The model under review builds one solid part; all positions refer to its coordinate system, in mm. Face numbers are marked on the shaded views. A direction names the side the tool comes from. Give positions to 0.01 mm unless a question says otherwise; leave off trailing zeros. Order: outer loops, then holes, each group sorted by start corner. A loop starts at its lowest first (then second) coordinate and runs counter-clockwise, first axis right, second up. Notation, with made-up numbers: (75, 83.5) - (122, 83.5) arc R12 cw to (122, 99.5) - close; hole circle Ø5 at (32, -23.5). An arc over 180 degrees is marked (long way). Put each result on its own line as item: value.
```python
from build123d import *

# Parameters (mm, degrees)
BOSS_EXTRUDE1_DEPTH = 8
SKETCH4_W           = 60
SKETCH4_H           = 30
BOSS_EXTRUDE2_DEPTH = 3
SKETCH5_R           = 3
CUT_EXTRUDE1_DEPTH  = 68.388900825
CUT_EXTRUDE3_DEPTH  = 61.736204501


# Read off the part's stored shape, not the designer's step: Boss-Extrude1
with BuildPart() as part:
    # Boss-Extrude1 outline → Boss-Extrude1 (new body)
    with BuildSketch(Plane.XY):
        with BuildLine():
            Line((-30, 0), (15, 0))
            add(Edge.make_bspline(
                [(15, 0), (15, -35), (-1.465594932, -45)],
                knots=[0, 0, 0, 1, 1, 1], degree=2))
            Line((-1.465594932, -45), (1.12987064, -49.273588476))
            add(Edge.make_bspline(
                [(20, 0), (20, -0.746108231), (19.988920633, -2.249243802), (19.922237871, -5.16766696), (19.754979798, -8.712103145), (19.418395555, -12.782160754), (18.785639236, -17.973362747), (17.643635897, -24.021456658), (15.683824621, -30.584336804), (13.095918314, -36.449845939), (8.74916419, -43.310162254), (4.437502248, -47.26477457), (1.12987064, -49.273588476)],
                knots=[0, 0, 0, 0, 0.03125, 0.0625, 0.125, 0.1875, 0.25, 0.375, 0.5, 0.625, 0.75, 1, 1, 1, 1], degree=3))
            Line((20, 0), (30, 0))
            Line((30, 0), (30, 5))
            Line((30, 5), (-30, 5))
            Line((-30, 5), (-30, 0))
        make_face()
    extrude(amount=BOSS_EXTRUDE1_DEPTH)

    # Sketch4 → Boss-Extrude2 (add)
    with BuildSketch(Plane(origin=(0, 5, 0), x_dir=(1, 0, 0), z_dir=(0, 1, 0))):
        with Locations((0, -4)):
            Rectangle(SKETCH4_W, SKETCH4_H)
    extrude(amount=BOSS_EXTRUDE2_DEPTH)

    # Sketch5 → Cut-Extrude1 (cut, through all)
    with BuildSketch(Plane(origin=(0, 8, 0), x_dir=(1, 0, 0), z_dir=(0, 1, 0))):
        with Locations(Location((25, -4, 0), (0, 0, 180))):
            Circle(SKETCH5_R)
    extrude(amount=-CUT_EXTRUDE1_DEPTH, mode=Mode.SUBTRACT)

    # Sketch7 → Cut-Extrude3 (cut, through all)
    with BuildSketch(Plane.XY.offset(8)):
        Polygon((-1.465594932, -45), (9.447885747, -41.814579425), (11.582932476, -49.129403534), (0.669451797, -52.314824109), align=None)
    extrude(amount=-CUT_EXTRUDE3_DEPTH, mode=Mode.SUBTRACT)


solid = part.part
```
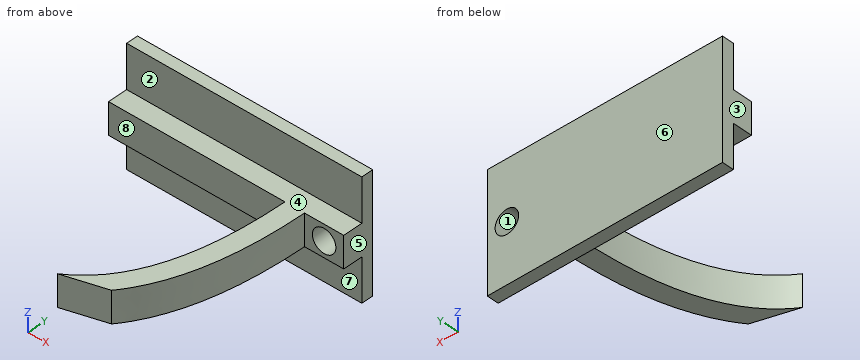
(1) The part is to be moulded in two halves that separate along X. For the marked faces 1, 2 and 3, say which applies: pulls with the +X half, pulls with the -X half, needs draft (parallel to the pull), parting line crosses it, or undercut.
The answers:
face 1: undercut
face 2: needs draft
face 3: pulls with the -X half
(2) Clearance check with flat-ended pins moving along their axes: pin 1 Ø25 at (x, y) = (10, -15.5) entering from +Z; pin 2 Ø3.5 at (x, z) = (2, -7) entering from -Y; pin 3 Ø2.5 at (x, z) = (-16.5, 2.5) entering from -Y. State where each tip first meets the part, or that it passes through.
The answers:
pin 1: z = 8
pin 2: y = 5
pin 3: y = 0
(3) Wall thickness on L1, parallel to Z at x = 25, y = 2.25; L2, parallel to Y at x = -8, z = 16; L3, parallel to X at y = 4, z = 3: over which ranges is each line inside the solid? List them lowest first.
The answers:
L1: 0 to 1, 7 to 8
L2: 5 to 8
L3: -30 to 22.17, 27.83 to 30
(4) For the marked faces 4, 5, 6, 7 and 8, list the 3-axis set-ups (+Z, -Z, +X, -X, +Y, -Y) from which the entire face can be reached by the end or side of a thin tool; tool diameter is ignored.
The answers:
face 4: +Z, +X, -X, -Y
face 5: +Z, -Z, +X, +Y, -Y
face 6: +Z, -Z, +X, -X, +Y
face 7: -Z, +X, -X, -Y
face 8: +Z, -Z, -X
(5) Take a section at C-C, the plane x = -3.5. Write out the cut boundary in (y, z), then the cut area to 3 significant figures.
The answers:
outline: (0, 0) - (5, 0) - (5, -11) - (8, -11) - (8, 19) - (5, 19) - (5, 8) - (0, 8) - close
area: 130 mm^2
(6) Take a section at B-B, the plane y = 3.5. Write out the cut boundary in (x, z).
The answers:
outline: (-30, 0) - (30, 0) - (30, 8) - (-30, 8) - close; hole circle Ø6 at (25, 4)
(7) Take a section at D-D, the plane z = -7.75. Write out the cut boundary in (x, y).
The answers:
outline: (-30, 5) - (30, 5) - (30, 8) - (-30, 8) - close
(8) Take a section at A-A, the plane x = 25. Write out the cut boundary in (y, z).
The answers:
outline: (0, 0) - (5, 0) - (5, -11) - (8, -11) - (8, 1) - (0, 1) - close; (0, 7) - (8, 7) - (8, 19) - (5, 19) - (5, 8) - (0, 8) - close
